from build123d import *

# Parameters (mm, degrees)
CROSS_DEPTH         = 4
BOTTOM_DEPTH        = 1
WALLS_DEPTH         = 1
WALLS_DEPTH_BACK    = 6
SKETCH5_W           = 6.9
SKETCH5_H           = 5
BOSS_EXTRUDE4_DEPTH = 4


with BuildPart() as part:
    # Sketch1 → Cross (new body)
    with BuildSketch(Plane(origin=(0, 0, 0), x_dir=(1, 0, 0), z_dir=(0, 1, 0))):
        Polygon((-0.8, 2.15), (0.8, 2.15), (0.8, 0.7), (2.15, 0.7), (2.15, -0.7), (0.8, -0.7), (0.8, -2.15), (-0.8, -2.15), (-0.8, -0.7), (-2.15, -0.7), (-2.15, 0.7), (-0.8, 0.7), align=None)
    extrude(amount=CROSS_DEPTH)

    # Sketch3 → Bottom (add)
    with BuildSketch(Plane.XZ):
        Polygon((10.478907386, 0), (5.239453693, 9.075), (-5.239453693, 9.075), (-10.478907386, 0), (-5.239453693, -9.075), (5.239453693, -9.075), align=None)
    extrude(amount=BOTTOM_DEPTH)

    # Sketch4 → Walls (add, two sides: drawn at the far end of the back side and taken through both)
    with BuildSketch(Plane.XZ.offset(-WALLS_DEPTH_BACK)):
        Polygon((5.816803962, -10.075), (11.633607924, 0), (5.816803962, 10.075), (-5.816803962, 10.075), (-11.633607924, 0), (-5.816803962, -10.075), align=None)
        Polygon((5.239453693, -9.075), (10.478907386, 0), (5.239453693, 9.075), (-5.239453693, 9.075), (-10.478907386, 0), (-5.239453693, -9.075), align=None, mode=Mode.SUBTRACT)
    extrude(amount=WALLS_DEPTH + WALLS_DEPTH_BACK)

    # Sketch5 → Boss-Extrude4 (add)
    with BuildSketch(Plane(origin=(0, 0, 0), x_dir=(1, 0, 0), z_dir=(0, 1, 0))):
        Polygon((8.054036255, 0), (4.027018128, 6.975), (-4.027018128, 6.975), (-8.054036255, 0), (-4.027018128, -6.975), (4.027018128, -6.975), align=None)
        Rectangle(SKETCH5_W, SKETCH5_H, mode=Mode.SUBTRACT)
    extrude(amount=BOSS_EXTRUDE4_DEPTH)


solid = part.part
Geometry check sheet. Reference: the model listing, model coordinates, mm. A direction names the side the tool comes from. Give positions to 0.01 mm unless a question says otherwise; leave off trailing zeros. Loops run counter-clockwise (first coordinate to the right, second up) from the corner with the lowest first, then second, coordinate; pieces in that order, holes last. Notation, with made-up numbers: M 45.25,39 L 49.25,39 A17 ccw 49.25,72 Z; hole C -40,21.5 d6. An arc over 180 degrees is marked long. Answer as a JSON object with one key per item and string values. Group by question number.
Item 1: Sectioned sample at B-B on y = 1.75. Give the number of separate pieces and of enclosed holes in the cut face, plus the area to 3 significant figures.
Item 2: Sectioned sample at D-D on z = 4.25. Record the boundary of the cut face in (x, y).
Item 3: Mould release check, pull along Z, two halves, no side actions. Record for faces 1 (the flat face through (9, 6, 4)), 2 (the flat face through (-2.15, 2, 0)), 3 (the flat face through (0, 3, -10.075)), 4 (the flat face through (-8.684, 2.549, 5.108)): pulls with the +Z half, pulls with the -Z half, needs draft (parallel to the pull), parting line crosses it, or undercut.
Item 4: Sectioned sample at C-C on x = 1.75. Record the boundary of the cut face in (y, z) (3 decimals), plus the area to 4 significant figures.
Item 5: Access from +Z, -Z, +X, -X, +Y, -Y to the whole of each face (thin tool, end or side, straight path). Record for faces 5 (the flat face through (3.45, 2, 0)), 6 (the flat face through (-8.766, 2.549, -4.967)).
Item 6: Sectioned sample at A-A on y = 4.75. Record the boundary of the cut face in (x, z) (3 decimals), plus the area to 3 significant figures.
Item 7: Gauge pin test, flat ends, axial feed: pin 1 (2 mm diameter, centred on x = -0.5, z = 0, fed in from +Y); pin 2 (0.7 mm diameter, centred on y = 2, z = 1, fed in from -X); pin 3 (1 mm diameter, centred on x = -6.5, y = 5.5, fed in from -Z); pin 4 (2 mm diameter, centred on x = -8.5, z = 8, fed in from +Y). Record the tip position at first contact, or that the pin passes through.
Item 8: Material ranges on L1, parallel to Z at x = 1.5, y = 3.75 (3 decimals); L2, parallel to Z at x = 0.75, y = 1.75 (3 decimals); L3, parallel to Z at x = -0.5, y = 5.25 (3 decimals), recorded low to high.
Findings below:
{
 "1": {"separate pieces": "3", "enclosed holes": "2", "area": "211 mm2"},
 "2": {"outline": "M -9.18,-1 L 9.18,-1 L 9.18,6 L 8.03,6 L 8.03,0 L 5.6,0 L 5.6,4 L -5.6,4 L -5.6,0 L -8.03,0 L -8.03,6 L -9.18,6 Z"},
 "3": {"face 1": "needs draft", "face 2": "undercut", "face 3": "pulls with the -Z half", "face 4": "pulls with the +Z half"},
 "4": {"outline": "M -1,-10.075 L 6,-10.075 L 6,-9.075 L 0,-9.075 L 0,-6.975 L 4,-6.975 L 4,-2.5 L 0,-2.5 L 0,-0.7 L 4,-0.7 L 4,0.7 L 0,0.7 L 0,2.5 L 4,2.5 L 4,6.975 L 0,6.975 L 0,9.075 L 6,9.075 L 6,10.075 L -1,10.075 Z", "area": "73.55 mm2"},
 "5": {"face 5": "+Y", "face 6": "-Z, -X, +Y, -Y"},
 "6": {"outline": "M -11.634,0 L -5.817,-10.075 L 5.817,-10.075 L 11.634,0 L 5.817,10.075 L -5.817,10.075 Z; hole M -10.479,0 L -5.239,-9.075 L 5.239,-9.075 L 10.479,0 L 5.239,9.075 L -5.239,9.075 Z", "area": "66.3 mm2"},
 "7": {"pin 1": "y = 4", "pin 2": "x = -11.26", "pin 3": "z = -9.76", "pin 4": "through"},
 "8": {"L1": "-10.075 to -9.075, -6.975 to -2.5, -0.7 to 0.7, 2.5 to 6.975, 9.075 to 10.075", "L2": "-10.075 to -9.075, -6.975 to -2.5, -2.15 to 2.15, 2.5 to 6.975, 9.075 to 10.075", "L3": "-10.075 to -9.075, 9.075 to 10.075"}
}
